Geometry: see drawing. Coordinates: mm, zero at the bounding-box minimum. Give positions to 0.01 mm unless a question says otherwise; leave off trailing zeros. Loops run counter-clockwise (first coordinate to the right, second up) from the corner with the lowest first, then second, coordinate; pieces in that order, holes last. Notation, with made-up numbers: M 65,84.5 L 116,84.5 A27 cw 116,108.5 Z; hole C -8,87 d10. An arc over 180 degrees is marked long. Answer in a Markdown table with one row per item.
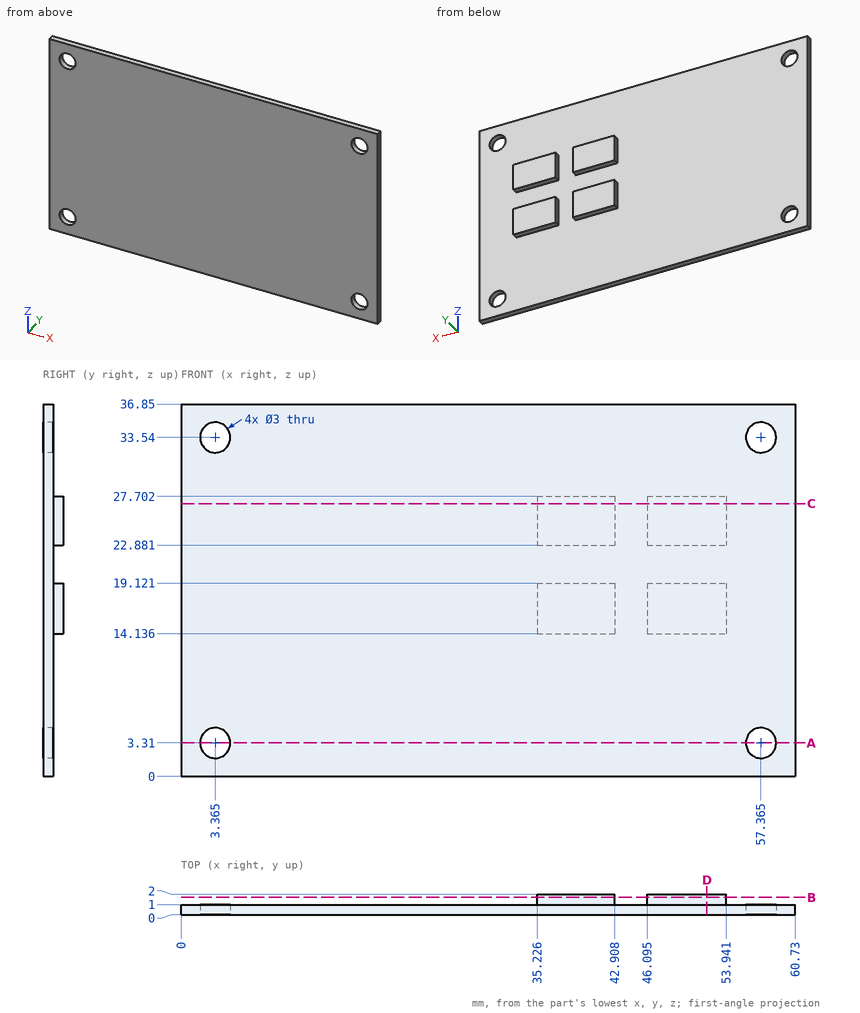
1) Section D-D, the plane x = 52. Return loops of the section in (y, z).
Reply:
| item | result |
|---|---|
| outline | M 0,0 L 1,0 L 1,14.14 L 2,14.14 L 2,19.12 L 1,19.12 L 1,22.88 L 2,22.88 L 2,27.7 L 1,27.7 L 1,36.85 L 0,36.85 Z |
2) Material intervals for L1, parallel to X at y = 0.7, z = 33.54 (1 decimal); L2, parallel to Z at x = 36, y = 1.95; L3, parallel to X at y = 1.6, z = 27 (1 decimal), sorted ascending.
Reply:
| item | result |
|---|---|
| L1 | x = 0 to 1.9, 4.9 to 55.9, 58.9 to 60.7 |
| L2 | z = 14.14 to 19.12, 22.88 to 27.7 |
| L3 | x = 35.2 to 42.9, 46.1 to 53.9 |
3) Section A-A, the plane z = 3.31. Return loops of the section in (x, y) (1 decimal).
Reply:
| item | result |
|---|---|
| outline | M 0,0 L 1.9,0 L 1.9,1 L 0,1 Z; M 4.9,0 L 55.9,0 L 55.9,1 L 4.9,1 Z; M 58.9,0 L 60.7,0 L 60.7,1 L 58.9,1 Z |
4) Section C-C, the plane z = 27. Return loops of the section in (x, y) (1 decimal).
Reply:
| item | result |
|---|---|
| outline | M 0,0 L 60.7,0 L 60.7,1 L 53.9,1 L 53.9,2 L 46.1,2 L 46.1,1 L 42.9,1 L 42.9,2 L 35.2,2 L 35.2,1 L 0,1 Z |
5) Pin query (flat end, axial travel): pin 1 Ø0.8 at (x, y) = (49, 1.5) entering from -Z; pin 2 Ø0.5 at (y, z) = (1.5, 17) entering from -X; pin 3 Ø1.1 at (y, z) = (1.5, 17) entering from +X; pin 4 Ø0.8 at (x, y) = (41, 1.5) entering from +Z. Return the tip coordinate at first contact, or that it passes through.
Reply:
| item | result |
|---|---|
| pin 1 | stops at z = 14.14 |
| pin 2 | stops at x = 35.23 |
| pin 3 | stops at x = 60.73 |
| pin 4 | stops at z = 27.7 |
6) Section B-B, the plane y = 1.7. Return loops of the section in (x, z) (1 decimal), then the cut area to 3 significant figures.
Reply:
| item | result |
|---|---|
| outline | M 35.2,14.1 L 42.9,14.1 L 42.9,19.1 L 35.2,19.1 Z; M 35.2,22.9 L 42.9,22.9 L 42.9,27.7 L 35.2,27.7 Z; M 46.1,14.1 L 53.9,14.1 L 53.9,19.1 L 46.1,19.1 Z; M 46.1,22.9 L 53.9,22.9 L 53.9,27.7 L 46.1,27.7 Z |
| area | 152 mm² |
